Can you work these out from the model? Positions are in its coordinate system, mm. Give positions to 0.01 mm unless a question says otherwise; leave off trailing zeros. Loops run counter-clockwise (first coordinate to the right, second up) from the corner with the lowest first, then second, coordinate; pieces in that order, holes last. Notation, with made-up numbers: M 55.5,64.5 L 82.5,64.5 A33 ccw 82.5,99.5 Z; hole C 57.5,75 d11. An arc over 180 degrees is marked long. Answer as a JSON object with one key per item and string values.
```python
from build123d import *

# Parameters (mm, degrees)
SKETCH1_R           = 1.25
BOSS_EXTRUDE1_DEPTH = 2.5
SKETCH2_R           = 1.25
BOSS_EXTRUDE2_DEPTH = 1.25


with BuildPart() as part:
    # Sketch1 → Boss-Extrude1 (new body)
    with BuildSketch(Plane(origin=(0, 0, 0), x_dir=(1, 0, 0), z_dir=(0, 1, 0))):
        with BuildLine():
            Line((-4, 0), (-4, 28))
            ThreePointArc((-4, 28), (0, 32), (4, 28))
            Line((4, 28), (4, 0))
            ThreePointArc((4, 0), (0, -4), (-4, 0))
        make_face()
        with Locations((0, 28)):
            Circle(SKETCH1_R, mode=Mode.SUBTRACT)
    extrude(amount=BOSS_EXTRUDE1_DEPTH)

    # Sketch2 → Boss-Extrude2 (add)
    with BuildSketch(Plane.XZ):
        Circle(SKETCH2_R)
    extrude(amount=BOSS_EXTRUDE2_DEPTH)


solid = part.part
```
1) Suppose I cut it at D-D, the plane x = 1.75. Write out the boundary of the cut face in (y, z), and give its area (3 significant figures).
Answer list:
{"outline": "M 0,-31.6 L 2.5,-31.6 L 2.5,3.6 L 0,3.6 Z", "area": "88.0 mm^2"}
2) Suppose I cut it at B-B, the plane y = 1.1. Write out the boundary of the cut face in (x, z).
Answer list:
{"outline": "M -4,-28 A4 ccw 4,-28 L 4,0 A4 ccw -4,0 Z; hole C 0,-28 d2.5"}
3) Suppose I cut it at A-A, the plane x = 0. Write out the boundary of the cut face in (y, z).
Answer list:
{"outline": "M -1.25,-1.25 L 0,-1.25 L 0,-26.75 L 2.5,-26.75 L 2.5,4 L 0,4 L 0,1.25 L -1.25,1.25 Z; M 0,-32 L 2.5,-32 L 2.5,-29.25 L 0,-29.25 Z"}
4) Will these pins go through, and if not, where does the flat tip stop? pin 1 Ø1.5 at (x, y) = (-2.5, 1) entering from +Z; pin 2 Ø4 at (x, z) = (-1.5, -16) entering from -Y.
Answer list:
{"pin 1": "z = 3.6", "pin 2": "y = 0"}
5) If we mould it in two halves opening along Z, with no side actions, what happens to faces 1 (the cylindrical face through (-0.27, 1.23, -26.78)), 2 (the flat face through (4, 1, -14)), 3 (the cylindrical face through (-0.27, -0.62, -1.22))? For each: +Z half, -Z half, draft (parallel to the pull), parting line (faces both ways), or undercut.
Answer list:
{"face 1": "undercut", "face 2": "draft", "face 3": "parting line"}
6) Suppose I cut it at C-C, the plane z = -5.5. Write out the boundary of the cut face in (x, y), and give its area (3 significant figures).
Answer list:
{"outline": "M -4,0 L 4,0 L 4,2.5 L -4,2.5 Z", "area": "20.0 mm^2"}
7) Please list where these lines run through material, in increasing order: line 1 along X through (y, z) = (0.8, -28); line 2 along Z through (x, y) = (0, 1.05); line 3 along Y through (x, z) = (2, 0). Write a range as from..to.
Answer list:
{"line 1": "-4..-1.25, 1.25..4", "line 2": "-32..-29.25, -26.75..4", "line 3": "0..2.5"}
